Part model, mm, in its own coordinate system. A direction names the side the tool comes from. Round coordinates to 2 decimals unless told otherwise and drop trailing zeros. Loops run counter-clockwise (first coordinate to the right, second up) from the corner with the lowest first, then second, coordinate; pieces in that order, holes last. Notation, with made-up numbers: M 62,43.25 L 116,43.25 A30 ccw 116,78.25 Z; hole C -18.5,71.5 d1. An arc over 180 degrees is marked long. Answer as CSV lines item,"result". Start each with the question number.
Item 1: Band-saw the part on D-D (z = -30.5). Give the cut face in (x, y), and give its area (3 significant figures).
Item 2: Band-saw the part on B-B (x = -40). Give the cut face in (y, z), and give its area (3 significant figures).
Item 3: Mould opens along X. For faces 5 (the flat face through (-12, 10, -1)), 6 (the flat face through (-7, 5, 5)), 7 (the flat face through (-18, 5, 52)) say: pulls with the +X half, pulls with the -X half, needs draft (parallel to the pull), parting line crosses it, or undercut.
Item 4: Drop flat-ended pins along their axis: pin 1 Ø5.5 at (y, z) = (8.5, 36.5) entering from -X; pin 2 Ø5 at (x, y) = (38.5, 3.5) entering from +Z; pin 3 Ø5 at (x, z) = (-40, 0) entering from -Y. Give the stop position or say it passes through.
Item 5: Which spindle directions (+Z, -Z, +X, -X, +Y, -Y) get a long thin tool onto all of the face, cutting with end or side? Do faces 1 (the cylindrical face through (16, 5, -9)), 2 (the cylindrical face through (42.53, 2.46, -1.61)), 3 (the flat face through (24.9, 4.9, 17.6)), 4 (the flat face through (-15, 2, -22.5)). Say none if no direction does.
Item 6: Wall check: line 1 (X direction, y = 7.45, z = -35); line 2 (X direction, y = 3.4, z = 0); line 3 (X direction, y = 6.3, z = 0). Give the ranges that are in metal, low to high.
Item 7: Band-saw the part on C-C (y = 2.5). Count the separate pieces of the cut face and the enclosed holes in it, and give its area (3 significant figures).
Item 8: Band-saw the part on A-A (z = 38.5). Give the cut face in (x, y).
```python
from build123d import *

# Parameters (mm, degrees)
SKETCH_1_R          = 1.6
SKETCH_1_R_2        = 1.35
EXTRUDE_1_DEPTH     = 10
SKETCH_2_R          = 3
CUT_EXTRUDE_1_DEPTH = 5
SKETCH_3_W          = 40
SKETCH_3_H          = 19
SKETCH_3_H_2        = 27.5
CUT_EXTRUDE_2_DEPTH = 5


with BuildPart() as part:
    # 草图1 → 凸台-拉伸1 (new body)
    with BuildSketch(Plane(origin=(0, 0, 0), x_dir=(1, 0, 0), z_dir=(0, 1, 0))):
        Polygon((-50, 7.5), (-50, -7.5), (-45, -12.5), (-30, -12.5), (-20, -22.5), (-20, -50), (-15, -55), (15, -55), (20, -50), (20, -22.5), (30, -12.5), (45, -12.5), (50, -7.5), (50, 7.5), (45, 12.5), (30, 12.5), (20, 22.5), (20, 50), (15, 55), (-15, 55), (-20, 50), (-20, 22.5), (-30, 12.5), (-45, 12.5), align=None)
        with Locations(Location((40, 0, 0), (0, 0, 270))):
            Circle(SKETCH_1_R, mode=Mode.SUBTRACT)
        with Locations(Location((-40, 0, 0), (0, 0, 270))):
            Circle(SKETCH_1_R, mode=Mode.SUBTRACT)
        with Locations(Location((-2, -50, 0), (0, 0, 270))):
            Circle(SKETCH_1_R_2, mode=Mode.SUBTRACT)
        with Locations(Location((-13.87, 5, 0), (0, 0, 270))):
            Circle(SKETCH_1_R_2, mode=Mode.SUBTRACT)
        with Locations(Location((26.13, 5, 0), (0, 0, 270))):
            Circle(SKETCH_1_R_2, mode=Mode.SUBTRACT)
        with Locations(Location((-13.87, 35, 0), (0, 0, 270))):
            Circle(SKETCH_1_R_2, mode=Mode.SUBTRACT)
        with BuildLine():
            Line((-6, 49), (6, 49))
            ThreePointArc((6, 49), (9.535533906, 47.535533906), (11, 44))
            Line((11, 44), (11, 24))
            ThreePointArc((11, 24), (9.535533906, 20.464466094), (6, 19))
            Line((6, 19), (-6, 19))
            ThreePointArc((-6, 19), (-9.535533906, 20.464466094), (-11, 24))
            Line((-11, 24), (-11, 44))
            ThreePointArc((-11, 44), (-9.535533906, 47.535533906), (-6, 49))
        make_face(mode=Mode.SUBTRACT)
        with BuildLine():
            Line((-9, -28), (7, -28))
            ThreePointArc((7, -28), (10.535533906, -29.464466094), (12, -33))
            Line((12, -33), (12, -42))
            ThreePointArc((12, -42), (10.535533906, -45.535533906), (7, -47))
            Line((7, -47), (-9, -47))
            ThreePointArc((-9, -47), (-12.535533906, -45.535533906), (-14, -42))
            Line((-14, -42), (-14, -33))
            ThreePointArc((-14, -33), (-12.535533906, -29.464466094), (-9, -28))
        make_face(mode=Mode.SUBTRACT)
        with BuildLine():
            Line((-2, 10), (13, 10))
            ThreePointArc((13, 10), (16.535533906, 8.535533906), (18, 5))
            Line((18, 5), (18, -15))
            ThreePointArc((18, -15), (16.535533906, -18.535533906), (13, -20))
            Line((13, -20), (-2, -20))
            ThreePointArc((-2, -20), (-5.535533906, -18.535533906), (-7, -15))
            Line((-7, -15), (-7, 5))
            ThreePointArc((-7, 5), (-5.535533906, 8.535533906), (-2, 10))
        make_face(mode=Mode.SUBTRACT)
    extrude(amount=EXTRUDE_1_DEPTH)

    # 草图2 → 切除-拉伸1 (cut)
    with BuildSketch(Plane.XZ):
        with Locations(Location((-40, 0, 0), (0, 0, 270))):
            Circle(SKETCH_2_R)
        with Locations(Location((40, 0, 0), (0, 0, 270))):
            Circle(SKETCH_2_R)
    extrude(amount=-CUT_EXTRUDE_1_DEPTH, mode=Mode.SUBTRACT)

    # 草图3 → 切除-拉伸2 (cut)
    with BuildSketch(Plane.XZ):
        with Locations((0, 37.5)):
            Rectangle(SKETCH_3_W, SKETCH_3_H)
        with Locations((0, -36.25)):
            Rectangle(SKETCH_3_W, SKETCH_3_H_2)
    extrude(amount=-CUT_EXTRUDE_2_DEPTH, mode=Mode.SUBTRACT)


solid = part.part
```
Answer block:
1,outline,"M -20,5 L -11,5 L -11,10 L -20,10 Z; M 11,5 L 20,5 L 20,10 L 11,10 Z"
1,area,"90.0 mm^2"
2,outline,"M 0,-12.5 L 10,-12.5 L 10,-1.6 L 5,-1.6 L 5,-3 L 0,-3 Z; M 0,3 L 5,3 L 5,1.6 L 10,1.6 L 10,12.5 L 0,12.5 Z"
2,area,"204 mm^2"
3,face 5,"needs draft"
3,face 6,"undercut"
3,face 7,"pulls with the -X half"
4,pin 1,"stops at x = -20"
4,pin 2,"stops at z = 12.5"
4,pin 3,"stops at y = 5"
5,face 1,"+Y, -Y"
5,face 2,"-Y"
5,face 3,"+Z, +X, +Y, -Y"
5,face 4,"+X, -X, -Y"
6,line 1,"x = -20 to -15.22, -12.52 to -11, 11 to 20"
6,line 2,"x = -50 to -43, -37 to -7, 18 to 37, 43 to 50"
6,line 3,"x = -50 to -41.6, -38.4 to -7, 18 to 38.4, 41.6 to 50"
7,separate pieces,"3"
7,enclosed holes,"6"
7,area,"3,270 mm^2"
8,outline,"M -20,5 L -14,5 L -14,10 L -20,10 Z; M 12,5 L 20,5 L 20,10 L 12,10 Z"
